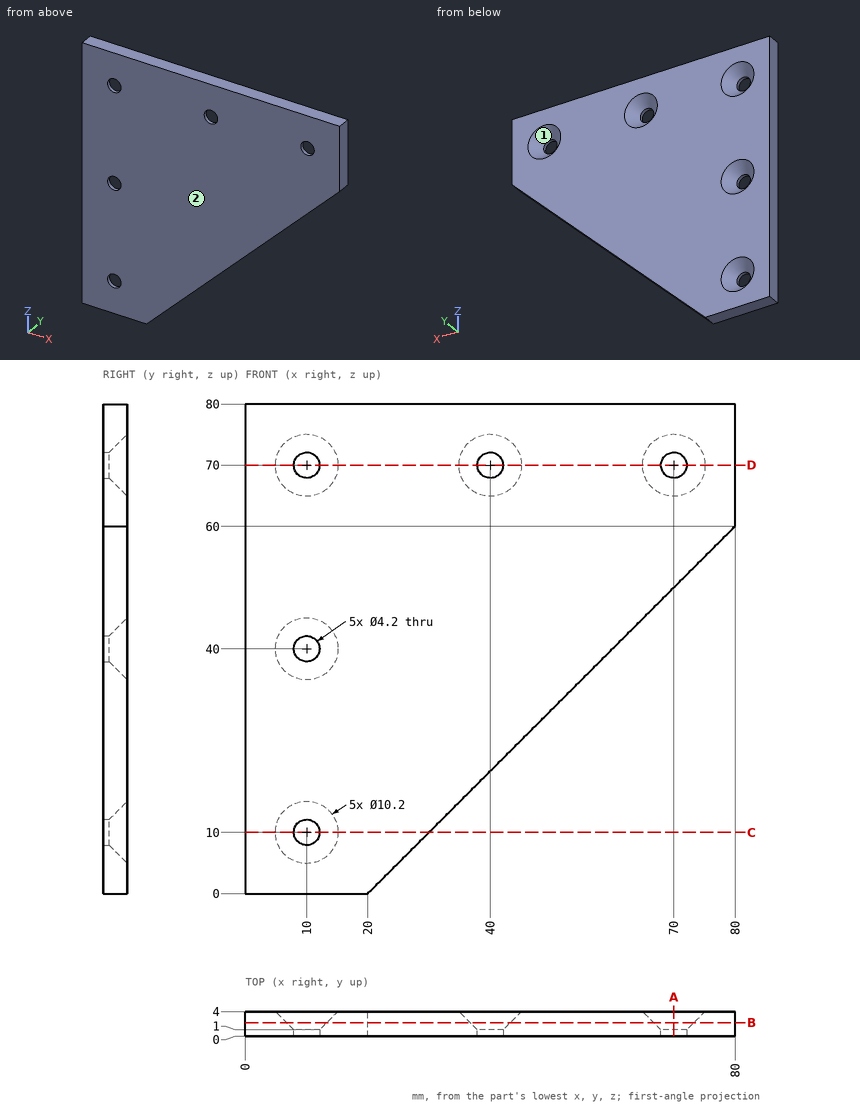
Geometry: see drawing. Coordinates: mm, zero at the bounding-box minimum. Give positions to 0.01 mm unless a question says otherwise; leave off trailing zeros. Loops run counter-clockwise (first coordinate to the right, second up) from the corner with the lowest first, then second, coordinate; pieces in that order, holes last. Notation, with made-up numbers: (75, 69) -> (132, 69) arc R13 ccw to (132, 74) -> close; hole circle Ø3 at (27.25, 80). An arc over 180 degrees is marked (long way). Use CSV: the item, a comma, the result in double quotes.
(1) Cut plane D-D (z = 70). Output: boundary loops of the cut face in (x, y).
From the geometry:
outline,"(0, 0) -> (7.9, 0) -> (7.9, 1) -> (4.9, 4) -> (0, 4) -> close; (12.1, 0) -> (37.9, 0) -> (37.9, 1) -> (34.9, 4) -> (15.1, 4) -> (12.1, 1) -> close; (42.1, 0) -> (67.9, 0) -> (67.9, 1) -> (64.9, 4) -> (45.1, 4) -> (42.1, 1) -> close; (72.1, 0) -> (80, 0) -> (80, 4) -> (75.1, 4) -> (72.1, 1) -> close"
(2) Cut plane A-A (x = 70). Output: boundary loops of the cut face in (y, z).
From the geometry:
outline,"(0, 50) -> (4, 50) -> (4, 64.9) -> (1, 67.9) -> (0, 67.9) -> close; (0, 72.1) -> (1, 72.1) -> (4, 75.1) -> (4, 80) -> (0, 80) -> close"
(3) First-contact query: P1, Ø1, axis at x = 68, z = 52.5, coming from the -Y side; P2, Ø5, axis at x = 10, z = 10, coming from the +Y side; P3, Ø1, axis at y = 3.5, z = 15.5, coming from the +X side; P4, Ø5.5, axis at x = 70, z = 70, coming from the +Y side. Flat tips, straight axial feed; report the tip coordinate or a pass-through.
From the geometry:
P1,"y = 0"
P2,"y = 1.4"
P3,"x = 36"
P4,"y = 1.65"
(4) Ray query, line 1 along X through (y, z) = (0.7, 70); line 2 along X through (y, z) = (0.65, 70.5). Return the intervals inside material, ascending. Write a range as [from, to].
From the geometry:
line 1,"[0, 7.9], [12.1, 37.9], [42.1, 67.9], [72.1, 80]"
line 2,"[0, 7.96], [12.04, 37.96], [42.04, 67.96], [72.04, 80]"
(5) Pull-direction query (Z, two-part tool) for the marked faces 1 and 2; classes: released by +Z, released by -Z, zero draft, split by the parting line, or undercut.
From the geometry:
face 1,"undercut"
face 2,"zero draft"
(6) Cut plane C-C (z = 10). Output: boundary loops of the cut face in (x, y), plus the area to 3 significant figures.
From the geometry:
outline,"(0, 0) -> (7.9, 0) -> (7.9, 1) -> (4.9, 4) -> (0, 4) -> close; (12.1, 0) -> (30, 0) -> (30, 4) -> (15.1, 4) -> (12.1, 1) -> close"
area,"94.2 mm^2"
(7) Cut plane B-B (y = 2.2). Output: boundary loops of the cut face in (x, z).
From the geometry:
outline,"(0, 0) -> (20, 0) -> (80, 60) -> (80, 80) -> (0, 80) -> close; hole circle Ø6.6 at (10, 10); hole circle Ø6.6 at (10, 40); hole circle Ø6.6 at (10, 70); hole circle Ø6.6 at (40, 70); hole circle Ø6.6 at (70, 70)"
